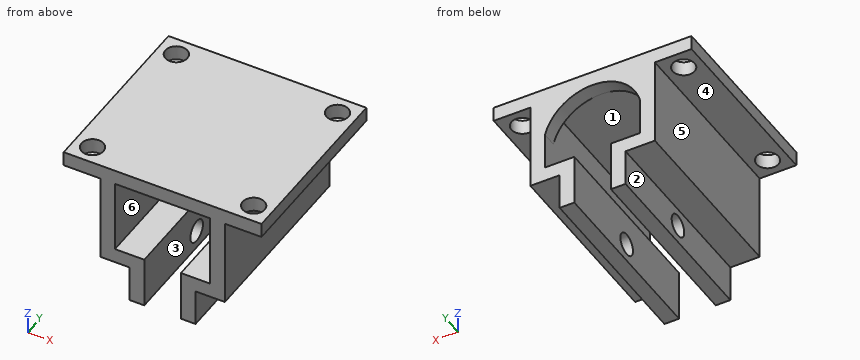
Solid Edge part; units mm, degrees
sketch "Sketch1" plane through (0, 0, 0) normal (0, -1, 0) x (1, 0, 0)
  line L0 (0, 10) -> (13.5, 10)
  line L1 (13.5, 10) -> (13.5, 8)
  line L2 (13.5, 8) -> (8.5, 8)
  line L3 (8.5, 8) -> (8.5, -4)
  line L4 (4.5, -4) -> (8.5, -4)
  line L5 (4.5, -9) -> (4.5, -4)
  line L6 (2.5, -9) -> (4.5, -9)
  line L7 (2.5, -2) -> (2.5, -9)
  line L8 (-2.5, -2) -> (2.5, -2)
  line L9 (-2.5, -9) -> (-2.5, -2)
  line L10 (-4.5, -9) -> (-2.5, -9)
  line L11 (-4.5, -4) -> (-4.5, -9)
  line L12 (-8.5, -4) -> (-4.5, -4)
  line L13 (-8.5, -4) -> (-8.5, 8)
  line L14 (-8.5, 8) -> (-13.5, 8)
  line L15 (-13.5, 8) -> (-13.5, 10)
  line L16 (-13.5, 10) -> (0, 10)
extrude "Protrusion1" add sketch "Sketch1" along normal blind 25
sketch "Sketch2" plane through (0, -25, 0.5) normal (0, -1, 0) x (1, 0, 0)
  line L0 (-6.5, 7.5) -> (-6.5, -2.5)
  line L1 (-6.5, -2.5) -> (6.5, -2.5)
  line L2 (6.5, -2.5) -> (6.5, 7.5)
  line L3 (6.5, 7.5) -> (-6.5, 7.5)
extrude "ExtrudedCutout_1" cut sketch "Sketch2" against normal blind 23
sketch "Sketch3" plane through (0, 0, 0.5) normal (0, 1, 0) x (-1, 0, 0)
  line L0 (-6.5, -2.5) -> (6.5, -2.5)
  line L1 (6.5, 2.5) -> (6.5, -2.5)
  arc A0 (0, 7.5) -> (6.5, 2.5) centre (0, 0.775) cw
  arc A1 (-6.5, 2.5) -> (0, 7.5) centre (0, 0.775) cw
  line L2 (-6.5, 2.5) -> (-6.5, -2.5)
extrude "ExtrudedCutout_2" cut sketch "Sketch3" against normal blind 2
sketch "Sketch4" plane through (0, -12.5, 10) normal (0, 0, 1) x (1, 0, 0)
  circle A0 centre (-11, 10) radius 1.5
  circle A1 centre (11, 10) radius 1.5
  circle A2 centre (11, -10) radius 1.5
  circle A3 centre (-11, -10) radius 1.5
extrude "Cutout1" cut sketch "Sketch4" against normal up to vertex (2 mm away)
sketch "Sketch5" plane through (4.5, -12.5, -6.5) normal (1, 0, 0) x (0, 1, 0)
  circle A0 centre (0, 0) radius 1.5
extrude "ExtrudedCutout_4" cut sketch "Sketch5" against normal blind 10.3838
For this review, take the finished solid that the model builds, in its own axes (mm). Face numbers are marked on the shaded views. A direction names the side the tool comes from. Give positions to 0.01 mm unless a question says otherwise; leave off trailing zeros. Order: outer loops, then holes, each group sorted by start corner. A loop starts at its lowest first (then second) coordinate and runs counter-clockwise, first axis right, second up. Notation, with made-up numbers: M 56.25,84 L 92.25,84 A22 cw 92.25,122 Z; hole C -23,5 d5. An arc over 180 degrees is marked long. Answer in a Markdown table with one row per item. Add a question column.
(1) Consider section B-B on z = -1. State the section outline as (x, y) points, and give its area (3 significant figures).
(2) For the marked faces 1, 2 and 3, list the 3-axis set-ups (+Z, -Z, +X, -X, +Y, -Y) from which the entire face can be reached by the end or side of a thin tool; tool diameter is ignored.
(3) Consider section D-D on y = -7. State the section outline as (x, z) points.
(4) Consider section A-A on y = -22.5. State the section outline as (x, z) points.
(5) Wall thickness on probe 1 along Z at (x, y) = (3.3, -12.5); probe 2 along Y at (x, z) = (-11, 8.65); probe 3 along X at (y, z) = (-22, 2.75): over which ranges is each line inside the solid? List them lowest first. Write a range as [from, to].
(6) For pin 1 (5 mm diameter, centred on y = -14.5, z = 2, fed in from -X); pin 2 (5.5 mm diameter, centred on x = -10, y = -18.5, fed in from -Z); pin 3 (2 mm diameter, centred on y = -16.5, z = -7, fed in from +X); pin 4 (5 mm diameter, centred on x = -9, z = -7, fed in from +Y), all flat-tipped, find the tip position at first contact; note any pin that passes through.
(7) Consider section C-C on x = 11. State the section outline as (y, z) points, and give its area (3 significant figures).
(8) Mouldability with a two-part tool opening along Z and no side actions: class the marked faces 4, 5 and 6 as +Z half, -Z half, draft (parallel to the pull), parting line (faces both ways), or undercut.
Evaluation:
| question | item | result |
|---|---|---|
| 1 | outline | M -8.5,-25 L -6.5,-25 L -6.5,0 L -8.5,0 Z; M 6.5,-25 L 8.5,-25 L 8.5,0 L 6.5,0 Z |
| 1 | area | 100 mm^2 |
| 2 | face 1 | -Y |
| 2 | face 2 | -Z, -X, +Y, -Y |
| 2 | face 3 | -Z, +Y, -Y |
| 3 | outline | M -13.5,8 L -8.5,8 L -8.5,-4 L -4.5,-4 L -4.5,-9 L -2.5,-9 L -2.5,-2 L -6.5,-2 L -6.5,8 L 6.5,8 L 6.5,-2 L 2.5,-2 L 2.5,-9 L 4.5,-9 L 4.5,-4 L 8.5,-4 L 8.5,8 L 13.5,8 L 13.5,10 L -13.5,10 Z |
| 4 | outline | M -13.5,8 L -12.5,8 L -12.5,10 L -13.5,10 Z; M -9.5,8 L -8.5,8 L -8.5,-4 L -4.5,-4 L -4.5,-9 L -2.5,-9 L -2.5,-2 L -6.5,-2 L -6.5,8 L 6.5,8 L 6.5,-2 L 2.5,-2 L 2.5,-9 L 4.5,-9 L 4.5,-4 L 8.5,-4 L 8.5,8 L 9.5,8 L 9.5,10 L -9.5,10 Z; M 12.5,8 L 13.5,8 L 13.5,10 L 12.5,10 Z |
| 5 | probe 1 | z = [-9, -8], [-5, -2], [8, 10] |
| 5 | probe 2 | y = [-25, -24], [-21, -4], [-1, 0] |
| 5 | probe 3 | x = [-8.5, -6.5], [6.5, 8.5] |
| 6 | pin 1 | stops at x = -8.5 |
| 6 | pin 2 | stops at z = -4 |
| 6 | pin 3 | stops at x = 4.5 |
| 6 | pin 4 | passes through |
| 7 | outline | M -25,8 L -24,8 L -24,10 L -25,10 Z; M -21,8 L -4,8 L -4,10 L -21,10 Z; M -1,8 L 0,8 L 0,10 L -1,10 Z |
| 7 | area | 38.0 mm^2 |
| 8 | face 4 | -Z half |
| 8 | face 5 | draft |
| 8 | face 6 | undercut |
